```python
from build123d import *

# Parameters (mm, degrees)
SKETCH1_R           = 0.95
BOSS_EXTRUDE1_DEPTH = 2.5
SKETCH2_R           = 0.95
BOSS_EXTRUDE2_DEPTH = 9.75
BOSS_EXTRUDE3_START = -1
SKETCH3_R           = 0.95
SKETCH3_R_2         = 2.75
BOSS_EXTRUDE3_DEPTH = 1
SKETCH4_R           = 1.75
SKETCH4_R_2         = 0.95
BOSS_EXTRUDE4_DEPTH = 1


with BuildPart() as part:
    # Sketch1 → Boss-Extrude1 (new body)
    with BuildSketch(Plane(origin=(0, 0, 0), x_dir=(1, 0, 0), z_dir=(0, 1, 0))):
        with BuildLine():
            Line((6.85, 5), (2.25, 5))
            Line((2.25, 5), (-2.25, 5))
            Line((-2.25, 5), (-6.85, 5))
            ThreePointArc((-6.85, 5), (-1.85, 0), (-6.85, -5))
            Line((-6.85, -5), (-2.35, -5))
            Line((-2.35, -5), (2.35, -5))
            Line((2.35, -5), (6.85, -5))
            ThreePointArc((6.85, -5), (1.85, 0), (6.85, 5))
        make_face()
        with Locations(Location((0, 0, 0), (0, 0, 270))):
            Circle(SKETCH1_R, mode=Mode.SUBTRACT)
    extrude(amount=BOSS_EXTRUDE1_DEPTH)

    # Sketch2 → Boss-Extrude2 (add)
    with BuildSketch(Plane(origin=(0, 0, 0), x_dir=(1, 0, 0), z_dir=(0, 1, 0))):
        with BuildLine():
            Line((-6.85, 5), (6.85, 5))
            ThreePointArc((6.85, 5), (11.85, 0), (6.85, -5))
            Line((6.85, -5), (-6.85, -5))
            ThreePointArc((-6.85, -5), (-11.85, 0), (-6.85, 5))
        make_face()
        with Locations(Location((0, 0, 0), (0, 0, 270))):
            Circle(SKETCH2_R, mode=Mode.SUBTRACT)
        with BuildLine():
            Line((-7.2, 3.984658078), (-7.2, 3.284658078))
            Line((-7.2, 3.284658078), (-6.5, 3.284658078))
            Line((-6.5, 3.284658078), (-6.5, 3.984658078))
            ThreePointArc((-6.5, 3.984658078), (-4.021572875, 2.828427125), (-2.865341922, 0.35))
            Line((-2.865341922, 0.35), (-3.565341922, 0.35))
            Line((-3.565341922, 0.35), (-3.565341922, -0.35))
            Line((-3.565341922, -0.35), (-2.865341922, -0.35))
            ThreePointArc((-2.865341922, -0.35), (-4.021572875, -2.828427125), (-6.5, -3.984658078))
            Line((-6.5, -3.984658078), (-6.5, -3.284658078))
            Line((-6.5, -3.284658078), (-7.2, -3.284658078))
            Line((-7.2, -3.284658078), (-7.2, -3.984658078))
            ThreePointArc((-7.2, -3.984658078), (-9.678427125, -2.828427125), (-10.834658078, -0.35))
            Line((-10.834658078, -0.35), (-10.134658078, -0.35))
            Line((-10.134658078, -0.35), (-10.134658078, 0.35))
            Line((-10.134658078, 0.35), (-10.834658078, 0.35))
            ThreePointArc((-10.834658078, 0.35), (-9.678427125, 2.828427125), (-7.2, 3.984658078))
        make_face(mode=Mode.SUBTRACT)
        with BuildLine():
            Line((-3.85, 4), (3.85, 4))
            ThreePointArc((3.85, 4), (2.532477728, 2.521706056), (1.892153285, 0.647885752))
            ThreePointArc((1.892153285, 0.647885752), (0, 2), (-1.892153285, 0.647885752))
            ThreePointArc((-1.892153285, 0.647885752), (-2.532477728, 2.521706056), (-3.85, 4))
        make_face(mode=Mode.SUBTRACT)
        with BuildLine():
            Line((-3.85, -4), (3.85, -4))
            ThreePointArc((3.85, -4), (2.532477728, -2.521706056), (1.892153285, -0.647885752))
            ThreePointArc((1.892153285, -0.647885752), (0, -2), (-1.892153285, -0.647885752))
            ThreePointArc((-1.892153285, -0.647885752), (-2.532477728, -2.521706056), (-3.85, -4))
        make_face(mode=Mode.SUBTRACT)
        with BuildLine():
            Line((6.5, 3.984658078), (6.5, 3.284658078))
            Line((6.5, 3.284658078), (7.2, 3.284658078))
            Line((7.2, 3.284658078), (7.2, 3.984658078))
            ThreePointArc((7.2, 3.984658078), (9.678427125, 2.828427125), (10.834658078, 0.35))
            Line((10.834658078, 0.35), (10.134658078, 0.35))
            Line((10.134658078, 0.35), (10.134658078, -0.35))
            Line((10.134658078, -0.35), (10.834658078, -0.35))
            ThreePointArc((10.834658078, -0.35), (9.678427125, -2.828427125), (7.2, -3.984658078))
            Line((7.2, -3.984658078), (7.2, -3.284658078))
            Line((7.2, -3.284658078), (6.5, -3.284658078))
            Line((6.5, -3.284658078), (6.5, -3.984658078))
            ThreePointArc((6.5, -3.984658078), (4.021572875, -2.828427125), (2.865341922, -0.35))
            Line((2.865341922, -0.35), (3.565341922, -0.35))
            Line((3.565341922, -0.35), (3.565341922, 0.35))
            Line((3.565341922, 0.35), (2.865341922, 0.35))
            ThreePointArc((2.865341922, 0.35), (4.021572875, 2.828427125), (6.5, 3.984658078))
        make_face(mode=Mode.SUBTRACT)
    extrude(amount=BOSS_EXTRUDE2_DEPTH)

    # Sketch3 → Boss-Extrude3 (add)
    with BuildSketch(Plane(origin=(0, 9.75, 0), x_dir=(1, 0, 0), z_dir=(0, 1, 0)).offset(BOSS_EXTRUDE3_START)):
        with BuildLine():
            Line((-6.85, 5), (6.85, 5))
            ThreePointArc((6.85, 5), (11.85, 0), (6.85, -5))
            Line((6.85, -5), (-6.85, -5))
            ThreePointArc((-6.85, -5), (-11.85, 0), (-6.85, 5))
        make_face()
        with Locations(Location((0, 0, 0), (0, 0, 270))):
            Circle(SKETCH3_R, mode=Mode.SUBTRACT)
        with Locations(Location((-6.85, 0, 0), (0, 0, 270))):
            Circle(SKETCH3_R_2, mode=Mode.SUBTRACT)
        with Locations(Location((6.85, 0, 0), (0, 0, 270))):
            Circle(SKETCH3_R_2, mode=Mode.SUBTRACT)
    extrude(amount=BOSS_EXTRUDE3_DEPTH)

    # Sketch4 → Boss-Extrude4 (add)
    with BuildSketch(Plane(origin=(0, 9.75, 0), x_dir=(1, 0, 0), z_dir=(0, 1, 0))):
        with Locations(Location((0, 0, 0), (0, 0, 270))):
            Circle(SKETCH4_R)
        with Locations(Location((0, 0, 0), (0, 0, 270))):
            Circle(SKETCH4_R_2, mode=Mode.SUBTRACT)
    extrude(amount=BOSS_EXTRUDE4_DEPTH)


solid = part.part
```
Can you work these out from the model? Positions are in its coordinate system, mm. A direction names the side the tool comes from. Round coordinates to 2 decimals unless told otherwise and drop trailing zeros. Loops run counter-clockwise (first coordinate to the right, second up) from the corner with the lowest first, then second, coordinate; pieces in that order, holes last. Notation, with made-up numbers: M 64.25,-16.75 L 78.25,-16.75 A3 ccw 78.25,-11.75 Z; hole C -6,-15.5 d6. An arc over 180 degrees is marked long. Answer in a Markdown table with one row per item.
1. On a 3-axis mill with a long thin cutter (end or side, diameter ignored), from which of +Z, -Z, +X, -X, +Y, -Y can I reach the whole of each face in a straight line? I mean faces 4 (the face through (0, 2.5, 3)), 5 (the face through (9.577, 9.243, -0.358)). Say none if no direction works.
Established:
| item | result |
|---|---|
| face 4 | none |
| face 5 | +Y, -Y |
2. If we section it at A-A, the plane x = 0: Please give me the cut outline in (y, z), plus the area to 3 significant figures.
Established:
| item | result |
|---|---|
| outline | M 0,-5 L 9.75,-5 L 9.75,-1.75 L 10.75,-1.75 L 10.75,-0.95 L 0,-0.95 Z; M 0,0.95 L 10.75,0.95 L 10.75,1.75 L 9.75,1.75 L 9.75,5 L 0,5 Z; hole M 2.5,-4 L 8.75,-4 L 8.75,-2 L 2.5,-2 Z; hole M 2.5,2 L 8.75,2 L 8.75,4 L 2.5,4 Z |
| area | 55.6 mm² |
3. If we section it at B-B, the plane z = -2.5: Please give me the cut outline in (x, y), plus the area to 3 significant figures.
Established:
| item | result |
|---|---|
| outline | M -11.18,0 L -9.97,0 L -9.97,8.75 L -8,8.75 L -8,9.75 L -11.18,9.75 Z; M -5.7,8.75 L -3.73,8.75 L -3.73,0 L 3.73,0 L 3.73,8.75 L 5.7,8.75 L 5.7,9.75 L -5.7,9.75 Z; M 8,8.75 L 9.97,8.75 L 9.97,0 L 11.18,0 L 11.18,9.75 L 8,9.75 Z; hole M -2.52,2.5 L 2.52,2.5 L 2.52,8.75 L -2.52,8.75 Z |
| area | 72.6 mm² |
4. If we section it at C-C, the plane y = 9: Please give me the cut outline in (x, z), plus the area to 3 significant figures.
Established:
| item | result |
|---|---|
| outline | M -6.85,-5 L 6.85,-5 A5 ccw 6.85,5 L -6.85,5 A5 ccw Z; hole C -6.85,0 d5.5; hole C 0,0 d1.9; hole C 6.85,0 d5.5 |
| area | 165 mm² |
5. I'm going to push flat-ended pins straight in: pin 1 Ø0.8 at (y, z) = (2.5, 3.5) entering from -X; pin 2 Ø0.8 at (y, z) = (6, -3.5) entering from +X; pin 3 Ø4 at (x, z) = (-7, 1) entering from +Y; pin 4 Ø5 at (x, z) = (-6, -3) entering from -Y. Where does each tip first touch, or does it pass through?
Established:
| item | result |
|---|---|
| pin 1 | x = -10.77 |
| pin 2 | x = 10.77 |
| pin 3 | y = 9.75 |
| pin 4 | y = 0 |
6. Thinking about a two-plate mould opening in X: for faces 1 (the face through (-2, 9.75, 0)), 2 (the face through (-4.049, 4.314, -2.856)), 3 (the face through (-1.71, 10.24, -0.38)), which applies, pulls with the +X half, pulls with the -X half, needs draft (parallel to the pull), parting line crosses it, or undercut?
Established:
| item | result |
|---|---|
| face 1 | needs draft |
| face 2 | undercut |
| face 3 | parting line crosses it |
7. Please list where these lines run through material, in increasing order: line 1 (X direction, y = 9.3, z = 0); line 2 (X direction, y = 4.5, z = 0); line 3 (Y direction, x = 1.25, z = 3.5). Write a range as from..to.
Established:
| item | result |
|---|---|
| line 1 | -11.85..-9.6, -4.1..-0.95, 0.95..4.1, 9.6..11.85 |
| line 2 | -11.85..-10.13, -3.57..-0.95, 0.95..3.57, 10.13..11.85 |
| line 3 | 0..2.5, 8.75..9.75 |
8. If we section it at D-D, the plane z = 0: Please give me the cut outline in (x, y).
Established:
| item | result |
|---|---|
| outline | M -11.85,0 L -10.13,0 L -10.13,8.75 L -9.6,8.75 L -9.6,9.75 L -11.85,9.75 Z; M -4.1,8.75 L -3.57,8.75 L -3.57,0 L -0.95,0 L -0.95,10.75 L -1.75,10.75 L -1.75,9.75 L -4.1,9.75 Z; M 0.95,0 L 3.57,0 L 3.57,8.75 L 4.1,8.75 L 4.1,9.75 L 1.75,9.75 L 1.75,10.75 L 0.95,10.75 Z; M 9.6,8.75 L 10.13,8.75 L 10.13,0 L 11.85,0 L 11.85,9.75 L 9.6,9.75 Z |
